```python
from build123d import *

# Parameters (mm, degrees)
IZIM1_R                     = 2
Y_KSEKLIK_EKSTR_ZYON1_DEPTH = 18
IZIM2_W                     = 29
IZIM2_H                     = 10
Y_KSEKLIK_EKSTR_ZYON2_DEPTH = 110
IZIM3_R                     = 2.05
KES_EKSTR_ZYON1_DEPTH       = 6
IZIM4_R                     = 2.05
KES_EKSTR_ZYON2_DEPTH       = 30
IZIM5_W                     = 6
IZIM5_H                     = 3
KES_EKSTR_ZYON3_DEPTH       = 9


with BuildPart() as part:
    # Çizim1 → Yükseklik-Ekstrüzyon1 (new body)
    with BuildSketch(Plane(origin=(0, 0, 0), x_dir=(1, 0, 0), z_dir=(0, 1, 0))):
        with BuildLine():
            Line((-39, 15), (-22, 15))
            ThreePointArc((-22, 15), (0, 3), (22, 15))
            Line((22, 15), (39, 15))
            Line((39, 15), (39, -20))
            Line((39, -20), (-39, -20))
            Line((-39, -20), (-39, 15))
        make_face()
        with Locations(Location((-29, 8, 0), (0, 0, 270))):
            Circle(IZIM1_R, mode=Mode.SUBTRACT)
        with Locations(Location((29, 8, 0), (0, 0, 270))):
            Circle(IZIM1_R, mode=Mode.SUBTRACT)
        with Locations(Location((-9.5, -12.5, 0), (0, 0, 270))):
            Circle(IZIM1_R, mode=Mode.SUBTRACT)
        with Locations(Location((9.5, -12.5, 0), (0, 0, 270))):
            Circle(IZIM1_R, mode=Mode.SUBTRACT)
    extrude(amount=Y_KSEKLIK_EKSTR_ZYON1_DEPTH)

    # Çizim2 → Yükseklik-Ekstrüzyon2 (add)
    with BuildSketch(Plane(origin=(0, 18, 0), x_dir=(1, 0, 0), z_dir=(0, 1, 0))):
        with Locations((-24.5, -2)):
            Rectangle(IZIM2_W, IZIM2_H)
        with Locations((24.5, -2)):
            Rectangle(IZIM2_W, IZIM2_H)
    extrude(amount=Y_KSEKLIK_EKSTR_ZYON2_DEPTH)

    # Çizim3 → Kes-Ekstrüzyon1 (cut)
    with BuildSketch(Plane(origin=(0, 18, 0), x_dir=(1, 0, 0), z_dir=(0, 1, 0))):
        with Locations(Location((-33, -13.5, 0), (0, 0, 270))):
            Circle(IZIM3_R)
        with Locations(Location((33, -13.5, 0), (0, 0, 90))):
            Circle(IZIM3_R)
    extrude(amount=-KES_EKSTR_ZYON1_DEPTH, mode=Mode.SUBTRACT)

    # Çizim4 → Kes-Ekstrüzyon2 (cut)
    with BuildSketch(Plane(origin=(0, 128, 0), x_dir=(1, 0, 0), z_dir=(0, 1, 0))):
        with Locations(Location((-24.5, -2, 0), (0, 0, 270))):
            Circle(IZIM4_R)
        with Locations(Location((24.5, -2, 0), (0, 0, 90))):
            Circle(IZIM4_R)
    extrude(amount=-KES_EKSTR_ZYON2_DEPTH, mode=Mode.SUBTRACT)

    # Çizim5 → Kes-Ekstrüzyon3 (cut)
    with BuildSketch(Plane(origin=(0, 0, -3), x_dir=(-1, 0, 0), z_dir=(0, 0, -1))):
        with Locations((24.5, 108)):
            Rectangle(IZIM5_W, IZIM5_H)
        with Locations((-24.5, 108)):
            Rectangle(IZIM5_W, IZIM5_H)
    extrude(amount=-KES_EKSTR_ZYON3_DEPTH, mode=Mode.SUBTRACT)


solid = part.part
```
Model file for the job. Use its own axes, mm. A direction names the side the tool comes from. Coordinates: 2 decimals unless noted, no trailing zeros. Write each loop counter-clockwise with the first axis right and the second up, starting at its lowest first coordinate (ties: lowest second). Pieces come first, ordered by that corner, then holes. Notation, with made-up numbers: (-34.75, -2) - (-26.75, -2) arc R17 ccw to (-26.75, 30) - close; hole circle Ø2 at (55, -35). An arc over 180 degrees is marked (long way). One line per question, with ' | ' between items. Start each with the question number.
Q1. Cut at B-B, the plane z = -1.5. List the corners of the cut face in (x, y).
Q2. Pin check, flat tips, straight feed: pin 1 (5 mm diameter, centred on x = -1, z = 14.5, fed in from +Y); pin 2 (0.9 mm diameter, centred on x = 24, y = 108, fed in from -Z); pin 3 (23 mm diameter, centred on x = -17.5, y = 79.5, fed in from -Z). Stop position of each tip, or through.
Q3. 3-axis set-ups, long thin cutter, end or side, ignore diameter. For faces 1 (the face through (-27.5, 108, 1)), 2 (the face through (24, 72, -3)), 3 (the face through (23.884, 118.88, 0.045)): which of +Z, -Z, +X, -X, +Y, -Y reach the whole face in a straight line?
Q4. Drill centre lines: line 1 (X direction, y = 103, z = 2); line 2 (X direction, y = 13.25, z = -8); line 3 (Z direction, x = 24.5, y = 123.25). Where is each one in solid material? Low to high. Write a range as [from, to].
Q5. Cut at C-C, the plane x = 33. List the corners of the cut face in (y, z).
Q6. Pull direction Y, two halves, no side cores. Call faces 4 (the face through (27.5, 108, 1)), 5 (the face through (1, 9, 20)), 6 (the face through (24.3, 128, -0.3)): pulls with the +Y half, pulls with the -Y half, needs draft (parallel to the pull), parting line crosses it, or undercut.
Q7. Cut at A-A, the plane y = 78. List the corners of the cut face in (x, z).
Q8. Cut at D-D, the plane x = 24.5. List the corners of the cut face in (y, z).
Answer below:
1) outline: (-39, 0) - (39, 0) - (39, 128) - (10, 128) - (10, 18) - (-10, 18) - (-10, 128) - (-39, 128) - close; hole (-27.5, 106.5) - (-21.5, 106.5) - (-21.5, 109.5) - (-27.5, 109.5) - close; hole (21.5, 106.5) - (27.5, 106.5) - (27.5, 109.5) - (21.5, 109.5) - close
2) pin 1: y = 18 | pin 2: z = 6 | pin 3: z = -3
3) face 1: -Z | face 2: -Z, +X, -X, +Y | face 3: +Y
4) line 1: [-39, -26.55], [-22.45, -10], [10, 22.45], [26.55, 39] | line 2: [-39, -31], [-27, -15.38], [15.38, 27], [31, 39] | line 3: [-3, -0.05], [4.05, 7]
5) outline: (0, -15) - (18, -15) - (18, -3) - (128, -3) - (128, 7) - (18, 7) - (18, 11.45) - (12, 11.45) - (12, 15.55) - (18, 15.55) - (18, 20) - (0, 20) - close
6) face 4: undercut | face 5: needs draft | face 6: pulls with the +Y half
7) outline: (-39, -3) - (-10, -3) - (-10, 7) - (-39, 7) - close; (10, -3) - (39, -3) - (39, 7) - (10, 7) - close
8) outline: (0, -15) - (18, -15) - (18, -3) - (106.5, -3) - (106.5, -0.05) - (98, -0.05) - (98, 4.05) - (106.5, 4.05) - (106.5, 6) - (109.5, 6) - (109.5, 4.05) - (128, 4.05) - (128, 7) - (18, 7) - (18, 20) - (0, 20) - close; (109.5, -3) - (128, -3) - (128, -0.05) - (109.5, -0.05) - close
